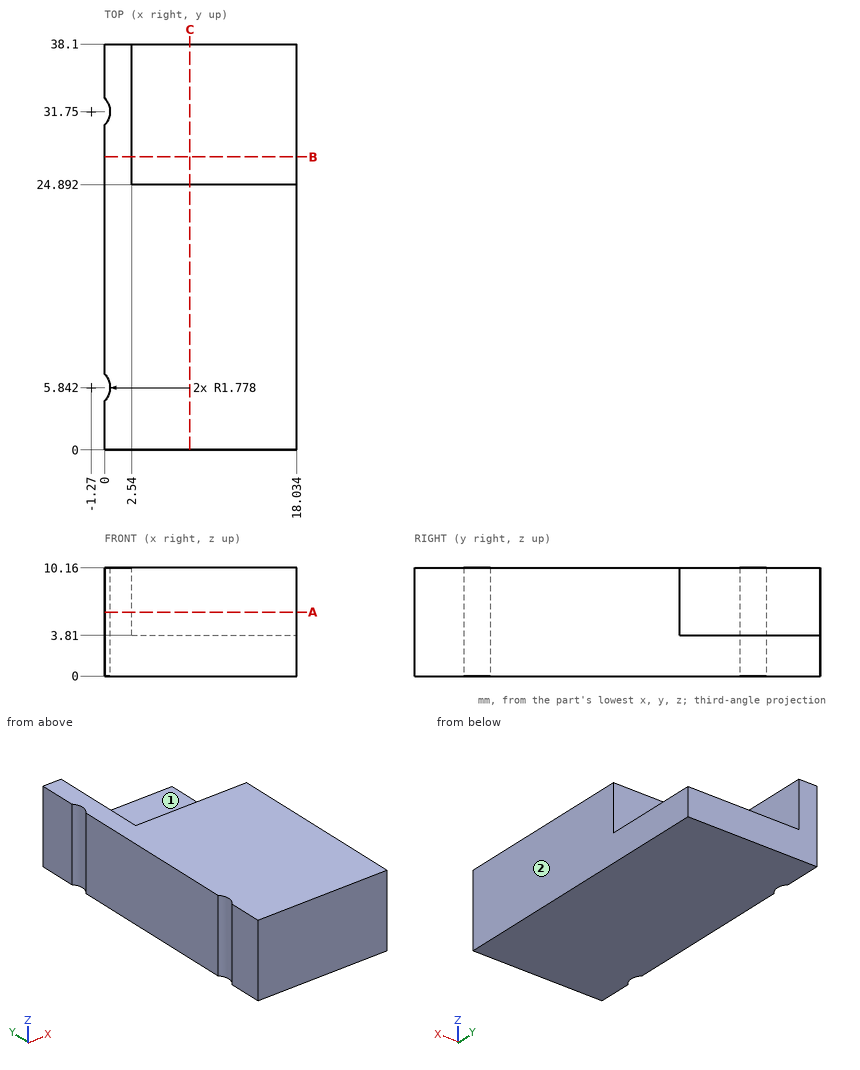
Check sheet for the drawn part. Datum: minimum x, y, z corner. Units: mm. A direction names the side the tool comes from. Round coordinates to 2 decimals unless told otherwise and drop trailing zeros. Order: outer loops, then holes, each group sorted by start corner. A loop starts at its lowest first (then second) coordinate and runs counter-clockwise, first axis right, second up. Notation, with made-up numbers: (-38.5, 12.25) -> (-27.5, 12.25) arc R22 ccw to (-27.5, 29.25) -> close; hole circle Ø9 at (56, 35). An arc over 180 degrees is marked (long way). Put each result on its own line as item: value.
1) Section check A-A (z = 6). Record the cut outline in (x, y), then the cut area to 3 significant figures.
Final values:
outline: (0, 0) -> (18.03, 0) -> (18.03, 24.89) -> (2.54, 24.89) -> (2.54, 38.1) -> (0, 38.1) -> (0, 32.99) arc R1.78 cw to (0, 30.51) -> (0, 7.09) arc R1.78 cw to (0, 4.6) -> close
area: 481 mm^2
2) Section check B-B (y = 27.5). Record the cut outline in (x, z), then the cut area to 3 significant figures.
Final values:
outline: (0, 0) -> (18.03, 0) -> (18.03, 3.81) -> (2.54, 3.81) -> (2.54, 10.16) -> (0, 10.16) -> close
area: 84.8 mm^2
3) Depth check by flat-ended pin: pin 1 (2 mm diameter, centred on x = 6.5, y = 32, fed in from +Z); pin 2 (5 mm diameter, centred on y = 32, z = 7.5, fed in from +X); pin 3 (5 mm diameter, centred on x = 13, z = 8, fed in from +Y). Enter the tip coordinate at first touch or a pass-through.
Final values:
pin 1: stops at z = 3.81
pin 2: stops at x = 2.54
pin 3: stops at y = 24.89
4) Section check C-C (x = 8). Record the cut outline in (y, z), then the cut area to 3 significant figures.
Final values:
outline: (0, 0) -> (38.1, 0) -> (38.1, 3.81) -> (24.89, 3.81) -> (24.89, 10.16) -> (0, 10.16) -> close
area: 303 mm^2
5) Material ranges on line 1 (Y direction, x = 8.25, z = 9); line 2 (Z direction, x = 8.5, y = 29.5); line 3 (X direction, y = 29, z = 5), recorded low to high.
Final values:
line 1: y = 0 to 24.89
line 2: z = 0 to 3.81
line 3: x = 0 to 2.54
6) Set-up check for the marked faces 1 and 2: record each of +Z, -Z, +X, -X, +Y, -Y from which the full face is reachable in a straight line by a thin tool's end or side.
Final values:
face 1: +Z, +X, +Y
face 2: +Z, -Z, +X, +Y, -Y
